from build123d import *

# Parameters (mm, degrees)
SKETCH1_R           = 10
BOSS_EXTRUDE1_DEPTH = 4
SKETCH2_R           = 15
BOSS_EXTRUDE2_DEPTH = 4
BOSS_EXTRUDE3_START = 20
SKETCH3_R           = 15
BOSS_EXTRUDE3_DEPTH = 20
SKETCH6_W           = 30
SKETCH6_H           = 5
CUT_EXTRUDE2_DEPTH  = 30.154759474
SKETCH7_R           = 5
CUT_EXTRUDE5_DEPTH  = 5


with BuildPart() as part:
    # Sketch1 → Boss-Extrude1 (new body)
    with BuildSketch(Plane(origin=(0, 0, 0), x_dir=(1, 0, 0), z_dir=(0, 1, 0))):
        with Locations(Location((0, 0, 0), (0, 0, 270))):
            Circle(SKETCH1_R)
    extrude(amount=-BOSS_EXTRUDE1_DEPTH)

    # Sketch2 → Boss-Extrude2 (add)
    with BuildSketch(Plane.XZ.offset(4)):
        with Locations(Location((0, 0, 0), (0, 0, 270))):
            Circle(SKETCH2_R)
    extrude(amount=BOSS_EXTRUDE2_DEPTH)

    # Sketch3 → Boss-Extrude3 (add)
    with BuildSketch(Plane(origin=(0, 0, 0), x_dir=(1, 0, 0), z_dir=(0, 1, 0)).offset(BOSS_EXTRUDE3_START)):
        with Locations(Location((0, 0, 0), (0, 0, 90))):
            Circle(SKETCH3_R)
    extrude(amount=-BOSS_EXTRUDE3_DEPTH)

    # Sketch6 → Cut-Extrude2 (cut, through all)
    with BuildSketch(Plane(origin=(0, 0, 0), x_dir=(1, 0, 0), z_dir=(0, 1, 0))):
        with Locations((0, -2.5)):
            Rectangle(SKETCH6_W, SKETCH6_H)
    cut_extrude2 = extrude(amount=CUT_EXTRUDE2_DEPTH, mode=Mode.SUBTRACT)

    # Sketch7 → Cut-Extrude5 (cut)
    with BuildSketch(Plane(origin=(0, 0, 5), x_dir=(-1, 0, 0), z_dir=(0, 0, -1))):
        with Locations((0, 13)):
            Circle(SKETCH7_R)
    cut_extrude5 = extrude(amount=-CUT_EXTRUDE5_DEPTH, mode=Mode.SUBTRACT)

    # Mirror1: Cut-Extrude2, Cut-Extrude5 across plane
    add(cut_extrude2.mirror(Plane.XY), mode=Mode.SUBTRACT)
    add(cut_extrude5.mirror(Plane.XY), mode=Mode.SUBTRACT)


solid = part.part
Model file for the job. Use its own axes, mm. A direction names the side the tool comes from. Coordinates: 2 decimals unless noted, no trailing zeros. Loops run counter-clockwise (first coordinate to the right, second up) from the corner with the lowest first, then second, coordinate; pieces in that order, holes last. Notation, with made-up numbers: (18.5, -32) -> (63.5, -32) arc R10 ccw to (63.5, -16) -> close; hole circle Ø10 at (19.25, 86.25). An arc over 180 degrees is marked (long way). Use one line per item in the form item = value. Start each with the question number.
(1) Cut at B-B on z = 11.5. Give the cut face in (x, y), and give its area (3 significant figures).
(2) Pull direction Y, two halves, no side cores. Call faces 1 (the flat face through (-10, -4, -3)), 2 (the cylindrical face through (0, 10, 15)), 3 (the flat face through (0, 13, -10)), 4 (the flat face through (0, -8, 0)): pulls with the +Y half, pulls with the -Y half, needs draft (parallel to the pull), parting line crosses it, or undercut.
(3) Flat gauge pins, fed straight in: pin 1 (8 mm diameter, centred on y = 6.5, z = -2, fed in from -X); pin 2 (3 mm diameter, centred on x = 2, z = 1, fed in from +Y); pin 3 (5 mm diameter, centred on x = 10, y = 1.5, fed in from -Z). Where does each tip first touch, or does it go through?
(4) Cut at C-C on x = -3.5. Give the cut face in (y, z).
(5) Cut at D-D on z = -8. Give the cut face in (x, y), and give its area (3 significant figures).
(6) Tool access for faces 5 (the flat face through (0, 20, 9)), 6 (the flat face through (0, 0, -11)), 7 (the flat face through (0, 0, 0)), 8 (the flat face through (0, 0, 11)), 9 (the cylindrical face through (0.651, 17.957, -7.465)): list every direction of +Z, -Z, +X, -X, +Y, -Y with a clear straight run to the whole face (end or side of a thin tool).
(7) Probe probe 1 along Y at (x, z) = (4.5, 12); probe 2 along Y at (x, z) = (0, 6.5); probe 3 along Z at (x, y) = (5, 16.25). List the from-to ranges inside material, lowest first. Write a range as from..to.
(8) Cut at A-A on y = 12.25. Give the cut face in (x, z).
Values:
q1.outline = (-9.63, -8) -> (9.63, -8) -> (9.63, -4) -> (-9.63, -4) -> close; (-9.63, 0) -> (9.63, 0) -> (9.63, 20) -> (-9.63, 20) -> close
q1.area = 462 mm2
q2.face_1 = undercut
q2.face_2 = needs draft
q2.face_3 = undercut
q2.face_4 = pulls with the -Y half
q3.pin_1 = -14.14
q3.pin_2 = 0
q3.pin_3 = -12.99
q4.outline = (-8, -14.59) -> (-4, -14.59) -> (-4, -9.37) -> (0, -9.37) -> (0, -14.59) -> (20, -14.59) -> (20, -5) -> (16.57, -5) -> (16.57, -10) -> (9.43, -10) -> (9.43, -5) -> (0, -5) -> (0, 5) -> (9.43, 5) -> (9.43, 10) -> (16.57, 10) -> (16.57, 5) -> (20, 5) -> (20, 14.59) -> (0, 14.59) -> (0, 9.37) -> (-4, 9.37) -> (-4, 14.59) -> (-8, 14.59) -> close
q5.outline = (-12.69, -8) -> (12.69, -8) -> (12.69, -4) -> (6, -4) -> (6, 0) -> (12.69, 0) -> (12.69, 20) -> (-12.69, 20) -> (-12.69, 0) -> (-6, 0) -> (-6, -4) -> (-12.69, -4) -> close; hole circle Ø10 at (0, 13)
q5.area = 579 mm2
q6.face_5 = +Z, -Z, +X, -X, +Y
q6.face_6 = -Z
q6.face_7 = +X, -X, +Y
q6.face_8 = +Z
q6.face_9 = none
q7.probe_1 = -8..-4, 0..20
q7.probe_2 = -8..8, 18..20
q7.probe_3 = -14.14..-5, 5..14.14
q8.outline = (-14.14, -5) arc R15 ccw to (14.14, -5) -> (4.94, -5) -> (4.94, -10) -> (-4.94, -10) -> (-4.94, -5) -> close; (-14.14, 5) -> (-4.94, 5) -> (-4.94, 10) -> (4.94, 10) -> (4.94, 5) -> (14.14, 5) arc R15 ccw to start
